Model file for the job. Use its own axes, mm. A direction names the side the tool comes from. Coordinates: 2 decimals unless noted, no trailing zeros. Order: outer loops, then holes, each group sorted by start corner. A loop starts at its lowest first (then second) coordinate and runs counter-clockwise, first axis right, second up. Notation, with made-up numbers: (38.25, 54.25) -> (70.25, 54.25) arc R17 cw to (70.25, 64.25) -> close; hole circle Ø4 at (-2.5, 28.25). An arc over 180 degrees is marked (long way). Return JSON: item names as keys, results as strings. Group by question number.
1) Which spindle directions (+Z, -Z, +X, -X, +Y, -Y) get a long thin tool onto all of the face, cutting with end or side? Do faces 1 (the flat face through (0, 0.5, 8)), 2 (the flat face through (0, -1, 0)). Say none if no direction does.
2) Probe line 1 (Y direction, x = 1.05, z = 9.25); line 2 (Z direction, x = 0.4, y = -3.5); line 3 (Y direction, x = -1, z = 3.25). List the from-to ranges inside material, lowest first.
3) Cut at C-C (z = 7.75). Write the cut outline in (x, y), and give its area (3 significant figures).
4) Cut at B-B (y = -3). Write the cut outline in (x, z), and give its area (3 significant figures).
5) Cut at D-D (x = -0.8). Write the cut outline in (y, z).
6) Cut at A-A (x = 0). Write the cut outline in (y, z), and give its area (3 significant figures).
7) Flat gauge pin, fed straight in: pin 1 (1.5 mm diameter, centred on x = -0.5, z = 10, fed in from -Y). Where does the tip first touch, or does it go through?
from build123d import *

# Parameters (mm, degrees)
BOSS_EXTRUDE1_DEPTH = 6
SKETCH1_3_W         = 3
SKETCH1_3_H         = 3
BOSS_EXTRUDE2_DEPTH = 11


with BuildPart() as part:
    # Sketch1 → Boss-Extrude1 (new body)
    with BuildSketch(Plane.XY):
        with BuildLine():
            Line((1.5, 0.5), (-1.5, 0.5))
            Line((-1.5, 0.5), (-1.5, -3.5))
            ThreePointArc((-1.5, -3.5), (0, -5), (1.5, -3.5))
            Line((1.5, -3.5), (1.5, 0.5))
        make_face()
    extrude(amount=BOSS_EXTRUDE1_DEPTH)

    # Sketch1<3> → Boss-Extrude2 (add)
    with BuildSketch(Plane.XY):
        with Locations((0, 2)):
            Rectangle(SKETCH1_3_W, SKETCH1_3_H)
    extrude(amount=BOSS_EXTRUDE2_DEPTH)


solid = part.part
Answers below:
{
 "1": {"face 1": "+Z, +X, -X, -Y", "face 2": "-Z, +X, -X, +Y, -Y"},
 "2": {"line 1": "y = 0.5 to 3.5", "line 2": "z = 0 to 6", "line 3": "y = -4.62 to 3.5"},
 "3": {"outline": "(-1.5, 0.5) -> (1.5, 0.5) -> (1.5, 3.5) -> (-1.5, 3.5) -> close", "area": "9.00 mm^2"},
 "4": {"outline": "(-1.5, 0) -> (1.5, 0) -> (1.5, 6) -> (-1.5, 6) -> close", "area": "18.0 mm^2"},
 "5": {"outline": "(-4.77, 0) -> (3.5, 0) -> (3.5, 11) -> (0.5, 11) -> (0.5, 6) -> (-4.77, 6) -> close"},
 "6": {"outline": "(-5, 0) -> (3.5, 0) -> (3.5, 11) -> (0.5, 11) -> (0.5, 6) -> (-5, 6) -> close", "area": "66.0 mm^2"},
 "7": {"pin 1": "stops at y = 0.5"}
}
